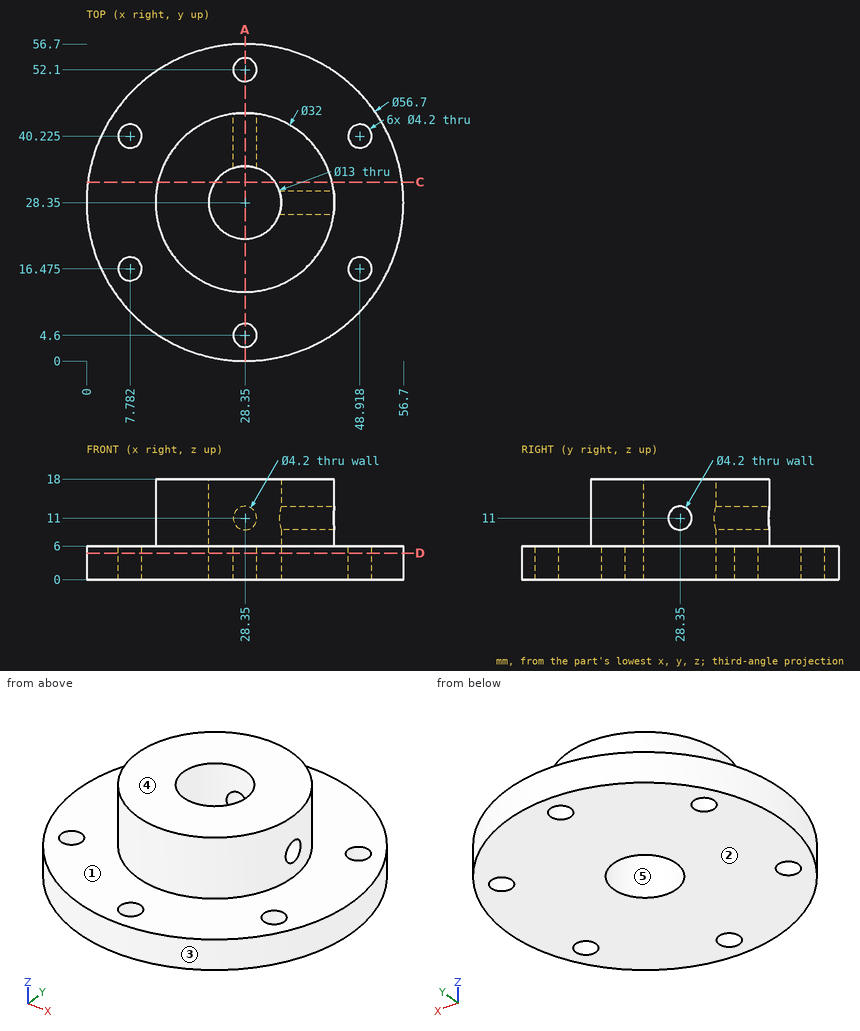
Source: three-view drawing plus pictorial views. Frame: mm from the lowest corner of the part. A direction names the side the tool comes from. Round coordinates to 2 decimals unless told otherwise and drop trailing zeros. Write each loop counter-clockwise with the first axis right and the second up, starting at its lowest first coordinate (ties: lowest second). Pieces come first, ordered by that corner, then holes. Notation, with made-up numbers: M -1,-12.5 L 53,-12.5 A10 cw 53,5.5 Z; hole C 69.25,25 d2. An arc over 180 degrees is marked long. Use CSV: the item, a comma, the result in double quotes. Start each with the question number.
Q1. First-contact query: P1, Ø10, axis at y = 49, z = 2, coming from the +X side; P2, Ø8, axis at y = 17, z = 16, coming from the -X side; P3, Ø11.5, axis at x = 28.35, y = 28.35, coming from the -Z side; P4, Ø2, axis at x = 16, z = 16, coming from the -Y side. Flat tips, straight axial feed; report the tip coordinate or a pass-through.
Q2. Access query for the marked faces 1 and 2. Directions: +Z, -Z, +X, -X, +Y, -Y. A direction counts if a zero-diameter tool reaches every point of the face in a straight line with its end or side. Return the directions, or none.
Q3. Cut plane D-D on z = 4.75. Count the separate pieces of the cut face and the enclosed holes in it, plus the area to 3 significant figures.
Q4. Cut plane C-C on y = 32. Output: boundary loops of the cut face in (x, z).
Q5. Line query: line 1 (Y direction, x = 28.35, z = 2); line 2 (Z direction, x = 28.35, y = 41.25); line 3 (Y direction, x = 48, z = 3.25) (1 decimal). Output: solid intervals per line, ascending. Write a range as from..to.
Q6. Cut plane A-A on x = 28.35. Output: boundary loops of the cut face in (y, z).
Q7. Pull-direction query (Y, two-part tool) for the marked faces 3, 4 and 5; classes: +Y half, -Y half, draft (parallel to the pull), parting line (faces both ways), or undercut.
Results found:
1,P1,"x = 51.99"
1,P2,"x = 14.14"
1,P3,"through"
1,P4,"y = 17.07"
2,face 1,"+Z"
2,face 2,"-Z, +X, -X, +Y, -Y"
3,separate pieces,"1"
3,enclosed holes,"7"
3,area,"2,310 mm^2"
4,outline,"M 0.24,0 L 22.97,0 L 22.97,18 L 12.77,18 L 12.77,6 L 0.24,6 Z; M 33.73,0 L 56.46,0 L 56.46,6 L 43.93,6 L 43.93,18 L 33.73,18 Z"
5,line 1,"0..2.5, 6.7..21.85, 34.85..50, 54.2..56.7"
5,line 2,"0..8.9, 13.1..18"
5,line 3,"7.9..14.6, 18.4..38.3, 42.1..48.8"
6,outline,"M 0,0 L 2.5,0 L 2.5,6 L 0,6 Z; M 6.7,0 L 21.85,0 L 21.85,18 L 12.35,18 L 12.35,6 L 6.7,6 Z; M 34.85,0 L 50,0 L 50,6 L 44.35,6 L 44.35,8.9 L 34.85,8.9 Z; M 34.85,13.1 L 44.35,13.1 L 44.35,18 L 34.85,18 Z; M 54.2,0 L 56.7,0 L 56.7,6 L 54.2,6 Z"
7,face 3,"parting line"
7,face 4,"draft"
7,face 5,"undercut"
